from build123d import *

# Parameters (mm, degrees)
SKETCH1_W           = 3.429
SKETCH1_H           = 4.1656
SKETCH2_R           = 2.0828
BOSS_EXTRUDE1_DEPTH = 9.525
CUT_EXTRUDE1_DEPTH  = 2.678906
CHAMFER1_SIZE       = 0.27628549
CHAMFER2_SIZE       = 0.769555748
CHAMFER2_SIZE2      = 0.538848736


with BuildPart() as part:
    # Sketch1 → Revolve1 (revolve)
    with BuildSketch(Plane.XZ):
        with Locations((12.082710259, 4.5828)):
            Rectangle(SKETCH1_W, SKETCH1_H)
    revolve(axis=Axis((10.368210259, 0, 6.6656), (0, 0, -1)))

    # Sketch2 → Boss-Extrude1 (add)
    with BuildSketch(Plane(origin=(0, 0, 2.5), x_dir=(-1, 0, 0), z_dir=(0, 0, -1))):
        with Locations((-10.368210259, 0)):
            Circle(SKETCH2_R)
    extrude(amount=BOSS_EXTRUDE1_DEPTH)

    # Sketch3 → Cut-Extrude1 (cut)
    with BuildSketch(Plane(origin=(0, 0, 3.98669375), x_dir=(-1, 0, 0), z_dir=(0, 0, -1))):
        Polygon((-10.368210259, -2.062222993), (-8.582272759, -1.031111496), (-8.582272759, 1.031111496), (-10.368210259, 2.062222993), (-12.154147759, 1.031111496), (-12.154147759, -1.031111496), align=None)
    extrude(amount=-CUT_EXTRUDE1_DEPTH, mode=Mode.SUBTRACT)

    # Chamfer1
    chamfer1_edges = [part.edges().sort_by_distance(p)[0] for p in [
        (6.939210259, 0, 2.5),
        (6.939210259, 0, 6.6656),
    ]]
    chamfer(chamfer1_edges, length=CHAMFER1_SIZE)

    # Chamfer2
    chamfer2_edges = [part.edges().sort_by_distance(p)[0] for p in [
        (12.451010259, 0, -7.025),
    ]]
    chamfer2_side = [part.faces().sort_by_distance(p)[0] for p in [
        (10.368210259, 0, -7.025),
    ]]
    chamfer(chamfer2_edges, length=CHAMFER2_SIZE, length2=CHAMFER2_SIZE2, reference=chamfer2_side[0])

    # Sketch4 → Cut-Revolve1 (revolve, cut)
    with BuildSketch(Plane(origin=(0, 0, 0), x_dir=(1, 0, 0), z_dir=(0, 1, 0))):
        Polygon((8.582272759, -6.38931451), (8.305987269, -6.6656), (8.582272759, -6.6656), align=None)
    revolve(axis=Axis((10.368210259, 0, 6.799545312), (0, 0, -1)), mode=Mode.SUBTRACT)


solid = part.part
Part model, mm, in its own coordinate system. A direction names the side the tool comes from. Give positions to 0.01 mm unless a question says otherwise; leave off trailing zeros. Loops run counter-clockwise (first coordinate to the right, second up) from the corner with the lowest first, then second, coordinate; pieces in that order, holes last.
(1) 3-axis set-ups, long thin cutter, end or side, ignore diameter. For faces 4 (the flat face through (10, 0, -7.025)), 5 (the flat face through (11.27, -1.54, 5.31)), 6 (the flat face through (8, 1, 2.5)): which of +Z, -Z, +X, -X, +Y, -Y reach the whole face in a straight line?
Return value:
face 4: -Z, +X, -X, +Y, -Y
face 5: +Z
face 6: -Z
(2) Band-saw the part on C-C (z = 1.25). Write the cut outline in (x, y).
Return value:
outline: circle Ø4.17 at (10.37, 0)
(3) Pin check, flat tips, straight feed: pin 1 (1.5 mm diameter, centred on x = 12.5, z = -4, fed in from -Y); pin 2 (1.5 mm diameter, centred on y = -1.5, z = 3.5, fed in from +X); pin 3 (3 mm diameter, centred on x = 10.5, y = 0.5, fed in from +Z). Stop position of each tip, or through.
Return value:
pin 1: stops at y = -1.56
pin 2: stops at x = 13.71
pin 3: stops at z = 6.62
(4) Pull direction X, two halves, no side cores. Call faces 1 (the flat face through (8, 1, 6.666)), 2 (the flat face through (9.46, 1.54, 5.31)), 3 (the cylindrical face through (8.382, 0.626, -1.93)): pulls with the +X half, pulls with the -X half, needs draft (parallel to the pull), parting line crosses it, or undercut.
Return value:
face 1: needs draft
face 2: undercut
face 3: parting line crosses it
(5) Band-saw the part on A-A (z = 5.5). Write the cut outline in (x, y), and give its area (3 significant figures).
Return value:
outline: circle Ø6.86 at (10.37, 0); hole (8.58, -1.03) - (10.37, -2.06) - (12.15, -1.03) - (12.15, 1.03) - (10.37, 2.06) - (8.58, 1.03) - close
area: 25.9 mm2
(6) Drill centre lines: line 1 along Z through (x, y) = (11, 0.5) (3 decimals); line 2 along Y through (x, z) = (10.5, 4.75); line 3 along Z through (x, y) = (9.5, -2.25). Where is each one in solid material? Low to high.
Return value:
line 1: z = -7.025 to 3.987
line 2: y = -3.43 to -1.99, 1.99 to 3.43
line 3: z = 2.5 to 6.67
